from build123d import *

# Parameters (mm, degrees)
SKETCH1_R                 = 19.75
SKETCH1_R_2               = 18.75
BOSS_EXTRUDE1_DEPTH       = 6
BOSS_EXTRUDE2_DEPTH       = 1
BOSS_EXTRUDE3_DEPTH       = 70
SKETCH4_R                 = 2.25
SKETCH4_R_2               = 1
BOSS_EXTRUDE4_DEPTH       = 21.5
SKETCH5_R                 = 1
BOSS_EXTRUDE5_DEPTH       = 22.5
SKETCH6_R                 = 2.25
SKETCH6_R_2               = 1
BOSS_EXTRUDE6_DEPTH       = 21.5
SKETCH7_R                 = 1
BOSS_EXTRUDE7_DEPTH       = 22.5
SKETCH8_R                 = 1
BOSS_EXTRUDE8_DEPTH       = 20
SKETCH9_R                 = 2.25
SKETCH9_R_2               = 1
BOSS_EXTRUDE9_DEPTH       = 18.5
SKETCH10_W                = 33
SKETCH10_H                = 53.5
BOSS_EXTRUDE10_DEPTH      = 22.5
BOSS_EXTRUDE11_DEPTH      = 12
BOSS_EXTRUDE11_DEPTH_BACK = 40
SKETCH11_W                = 38
SKETCH11_H                = 38
SKETCH12_R                = 16
BOSS_EXTRUDE12_DEPTH      = 3


with BuildPart() as part:
    # Sketch1 → Boss-Extrude1 (new body)
    with BuildSketch(Plane.XY):
        Circle(SKETCH1_R)
        Circle(SKETCH1_R_2, mode=Mode.SUBTRACT)
    extrude(amount=BOSS_EXTRUDE1_DEPTH)

    # Sketch2 → Boss-Extrude2 (add)
    with BuildSketch(Plane(origin=(0, 0, 0), x_dir=(-1, 0, 0), z_dir=(0, 0, -1))):
        with BuildLine():
            ThreePointArc((-12.464487037, 16.589124838), (-20.75, 0), (-12.464487037, -16.589124838))
            ThreePointArc((-12.464487037, -16.589124838), (-11.549423528, -20.004188348), (-8.134360018, -19.089124838))
            ThreePointArc((-8.134360018, -19.089124838), (10.375, -17.970027129), (20.598847055, -2.5))
            ThreePointArc((20.598847055, -2.5), (23.098847055, 0), (20.598847055, 2.5))
            ThreePointArc((20.598847055, 2.5), (10.375, 17.970027129), (-8.134360018, 19.089124838))
            ThreePointArc((-8.134360018, 19.089124838), (-11.549423528, 20.004188348), (-12.464487037, 16.589124838))
        make_face()
    extrude(amount=BOSS_EXTRUDE2_DEPTH)

    # Sketch3 → Boss-Extrude3 (add)
    with BuildSketch(Plane(origin=(0, 0, -1), x_dir=(-1, 0, 0), z_dir=(0, 0, -1))):
        with BuildLine():
            Line((16.007810594, 4), (18.5, 4))
            Line((18.5, 4), (18.5, -4))
            Line((18.5, -4), (16.007810594, -4))
            ThreePointArc((16.007810594, -4), (0, -16.5), (-16.007810594, -4))
            Line((-16.007810594, -4), (-18.5, -4))
            Line((-18.5, -4), (-18.5, 4))
            Line((-18.5, 4), (-16.007810594, 4))
            ThreePointArc((-16.007810594, 4), (0, 16.5), (16.007810594, 4))
        make_face()
    extrude(amount=BOSS_EXTRUDE3_DEPTH)

    # Sketch4 → Boss-Extrude4 (add, symmetric)
    with BuildSketch(Plane(origin=(0, 0, 0), x_dir=(1, 0, 0), z_dir=(0, 1, 0))):
        with Locations(Location((0, 13, 0), (0, 0, 90))):
            Circle(SKETCH4_R)
        with Locations(Location((0, 13, 0), (0, 0, 90))):
            Circle(SKETCH4_R_2, mode=Mode.SUBTRACT)
    extrude(amount=BOSS_EXTRUDE4_DEPTH, both=True)

    # Sketch5 → Boss-Extrude5 (add, symmetric)
    with BuildSketch(Plane(origin=(0, 0, 0), x_dir=(1, 0, 0), z_dir=(0, 1, 0))):
        with Locations(Location((0, 9.5, 0), (0, 0, 90))):
            Circle(SKETCH5_R)
    extrude(amount=BOSS_EXTRUDE5_DEPTH, both=True)

    # Sketch6 → Boss-Extrude6 (add)
    with BuildSketch(Plane(origin=(0, 0, 0), x_dir=(1, 0, 0), z_dir=(0, 1, 0))):
        with Locations(Location((3, 50.5, 0), (0, 0, 270))):
            Circle(SKETCH6_R)
        with Locations(Location((3, 50.5, 0), (0, 0, 270))):
            Circle(SKETCH6_R_2, mode=Mode.SUBTRACT)
    extrude(amount=-BOSS_EXTRUDE6_DEPTH)

    # Sketch7 → Boss-Extrude7 (add)
    with BuildSketch(Plane(origin=(0, 0, 0), x_dir=(1, 0, 0), z_dir=(0, 1, 0))):
        with Locations(Location((0.5, 54.5, 0), (0, 0, 270))):
            Circle(SKETCH7_R)
    extrude(amount=-BOSS_EXTRUDE7_DEPTH)

    # Sketch8 → Boss-Extrude8 (add)
    with BuildSketch(Plane(origin=(0, 0, 0), x_dir=(0, 0, -1), z_dir=(1, 0, 0))):
        with Locations((20, 0)):
            Circle(SKETCH8_R)
    extrude(amount=-BOSS_EXTRUDE8_DEPTH)

    # Sketch9 → Boss-Extrude9 (add)
    with BuildSketch(Plane(origin=(0, 0, 0), x_dir=(0, 0, -1), z_dir=(1, 0, 0))):
        with Locations((20, 10)):
            Circle(SKETCH9_R)
        with Locations((20, 10)):
            Circle(SKETCH9_R_2, mode=Mode.SUBTRACT)
    extrude(amount=-BOSS_EXTRUDE9_DEPTH)

    # Sketch10 → Boss-Extrude10 (add)
    with BuildSketch(Plane(origin=(0, 0, 0), x_dir=(1, 0, 0), z_dir=(0, 1, 0))):
        with Locations((0, 51.75)):
            Rectangle(SKETCH10_W, SKETCH10_H)
    extrude(amount=BOSS_EXTRUDE10_DEPTH)

    # Sketch11 → Boss-Extrude11 (add, two sides: drawn at the far end of the back side and taken through both)
    with BuildSketch(Plane(origin=(0, 0, -71), x_dir=(-1, 0, 0), z_dir=(0, 0, -1)).offset(-BOSS_EXTRUDE11_DEPTH_BACK)):
        Rectangle(SKETCH11_W, SKETCH11_H)
    extrude(amount=BOSS_EXTRUDE11_DEPTH + BOSS_EXTRUDE11_DEPTH_BACK)

    # Sketch12 → Boss-Extrude12 (add)
    with BuildSketch(Plane.XY):
        with Locations(Location((0, 0, 0), (0, 0, 180))):
            Circle(SKETCH12_R)
    extrude(amount=BOSS_EXTRUDE12_DEPTH)


solid = part.part
For this review, take the finished solid that the model builds, in its own axes (mm). A direction names the side the tool comes from. Round coordinates to 2 decimals unless told otherwise and drop trailing zeros. Write each loop counter-clockwise with the first axis right and the second up, starting at its lowest first coordinate (ties: lowest second). Pieces come first, ordered by that corner, then holes. Notation, with made-up numbers: M -2.5,-6.75 L 13.5,-6.75 A19 ccw 13.5,-2.75 Z; hole C 41.25,67.5 d6. An arc over 180 degrees is marked long. Write item = value, one per line. Start each with the question number.
(1) The part is to be moulded in two halves that separate along X. For faces 5 (the face through (0, -16.5, -13)), 6 (the face through (-18.5, 9, -19)), 7 (the face through (0, 0, 3)), 8 (the face through (0, 22.5, -9)), say which applies: +X half, -X half, draft (parallel to the pull), parting line (faces both ways), or undercut.
(2) We need section A-A (z = -54.5). Give the boundary of the cut face in (x, y).
(3) For line 1 along Y through (x, z) = (0, 2); line 2 along Z through (x, y) = (-10.5, 16); line 3 along X through (y, z) = (-19.15, -13), list the stretches that pass through material, from the lowest coordinate up.
(4) We need section B-B (y = 14). Give the boundary of the cut face in (x, z).
(5) For faces 1 (the face through (-14.6, 13.3, 3)), 2 (the face through (0.6, -19.4, -8.7)), 3 (the face through (17, -4, -16)), 4 (the face through (-10.61, 17.83, -0.49)), list the 3-axis set-ups (+Z, -Z, +X, -X, +Y, -Y) from which the entire face can be reached by the end or side of a thin tool; tool diameter is ignored.
(6) We need section C-C (x = -8.5). Give the boundary of the cut face in (y, z), then the cut area to 3 significant figures.
(7) We need section D-D (z = -13). Give the boundary of the cut face in (x, y).
(8) Clearance check with flat-ended pins moving along their axes: pin 1 Ø3 at (x, z) = (-4, -27.5) entering from -Y; pin 2 Ø10 at (x, y) = (14.5, 11) entering from +Z; pin 3 Ø1.3 at (x, z) = (0, -12.5) entering from +Y; pin 4 Ø8 at (y, z) = (-2, -39.5) entering from +X. State where each tip first meets the part, or that it passes through.
Results found:
q1.face_5 = undercut
q1.face_6 = -X half
q1.face_7 = undercut
q1.face_8 = draft
q2.outline = M -19,-19 L -0.5,-19 L -0.5,-22.5 L 1.5,-22.5 L 1.5,-19 L 19,-19 L 19,19 L 16.5,19 L 16.5,22.5 L -16.5,22.5 L -16.5,19 L -19,19 Z
q3.line_1 = -19.75 to -18.75, -16 to 16, 18.75 to 19.75
q3.line_2 = -83 to -25, -1 to 6
q3.line_3 = -2.25 to -1, 1 to 2.25
q4.outline = M -19,-83 L 19,-83 L 19,-31 L 16.5,-31 L 16.5,-25 L 8.73,-25 L 8.73,-1 L 15.32,-1 L 15.32,0 L 13.93,0 L 13.93,6 L 12.47,6 L 12.47,0 L 7.75,0 L 7.75,3 L -7.75,3 L -7.75,0 L -12.47,0 L -12.47,6 L -13.93,6 L -13.93,0 L -15.32,0 L -15.32,-1 L -8.73,-1 L -8.73,-25 L -16.5,-25 L -16.5,-31 L -19,-31 Z
q5.face_1 = +Z
q5.face_2 = -Y
q5.face_3 = +X, -Y
q5.face_4 = +Z, +Y
q6.outline = M -19,-83 L 19,-83 L 19,-78.5 L 22.5,-78.5 L 22.5,-25 L 14.14,-25 L 14.14,-1 L 18.93,-1 L 18.93,0 L 17.83,0 L 17.83,6 L 16.71,6 L 16.71,0 L 13.56,0 L 13.56,3 L -13.56,3 L -13.56,0 L -16.71,0 L -16.71,6 L -17.83,6 L -17.83,0 L -18.93,0 L -18.93,-1 L -14.14,-1 L -14.14,-31 L -19,-31 Z
q6.area = 3,170 mm²
q7.outline = M -18.5,-4 L -16.01,-4 A16.5 ccw -2.25,-16.35 L -2.25,-21.5 L -1,-21.5 L -1,-16.47 A16.5 ccw 1,-16.47 L 1,-21.5 L 2.25,-21.5 L 2.25,-16.35 A16.5 ccw 16.01,-4 L 18.5,-4 L 18.5,4 L 16.01,4 A16.5 ccw 2.25,16.35 L 2.25,21.5 L 1,21.5 L 1,16.47 A16.5 ccw -1,16.47 L -1,21.5 L -2.25,21.5 L -2.25,16.35 A16.5 ccw -16.01,4 L -18.5,4 Z
q8.pin_1 = -16.31
q8.pin_2 = 6
q8.pin_3 = 21.5
q8.pin_4 = 19
